```python
from build123d import *

# Parameters (mm, degrees)
SKETCH3_W           = 200
SKETCH3_H           = 50
BOSS_EXTRUDE2_DEPTH = 1
SKETCH4_R           = 2
BOSS_EXTRUDE3_DEPTH = 2


with BuildPart() as part:
    # Sketch3 → Boss-Extrude2 (new, symmetric)
    with BuildSketch(Plane(origin=(0, 0, 0), x_dir=(1, 0, 0), z_dir=(0, 1, 0))):
        Rectangle(SKETCH3_W, SKETCH3_H)
    extrude(amount=BOSS_EXTRUDE2_DEPTH, both=True)

    # Sketch4 → Boss-Extrude3 (add)
    # profile 1 of 2: a face of its own
    with BuildSketch(Plane.XY.offset(25)):
        with BuildLine():
            Line((100, -1), (90, -1))
            Line((90, -1), (90, 21))
            ThreePointArc((90, 21), (95, 26), (100, 21))
            Line((100, 21), (100, -1))
        make_face()
        with Locations((95, 21)):
            Circle(SKETCH4_R, mode=Mode.SUBTRACT)
    # profile 2 of 2: a face of its own
    with BuildSketch(Plane.XY.offset(25)):
        with BuildLine():
            Line((-90, -1), (-90, 21))
            ThreePointArc((-90, 21), (-95, 26), (-100, 21))
            Line((-100, 21), (-100, -1))
            Line((-100, -1), (-90, -1))
        make_face()
        with Locations(Location((-95, 21, 0), (0, 0, 180))):
            Circle(SKETCH4_R, mode=Mode.SUBTRACT)
    extrude(amount=BOSS_EXTRUDE3_DEPTH)


solid = part.part
```
Here's how the part is built. I have some questions about the finished solid (model axes, mm). A direction names the side the tool comes from. Round coordinates to 2 decimals unless told otherwise and drop trailing zeros. Write each loop counter-clockwise with the first axis right and the second up, starting at its lowest first coordinate (ties: lowest second). Pieces come first, ordered by that corner, then holes. Notation, with made-up numbers: M 21.5,-17 L 33.5,-17 A34 ccw 33.5,16 Z; hole C 52.25,88 d11. An arc over 180 degrees is marked long. Answer as CSV lines item,"result". Start each with the question number.
1. Suppose I cut it at D-D on z = 5. Write out the boundary of the cut face in (x, y), then the cut area to 3 significant figures.
2. Suppose I cut it at A-A on y = 15. Write out the boundary of the cut face in (x, z).
3. Thinking about a two-plate mould opening in X: for faces 3 (the cylindrical face through (96.908, 21.601, 25.986)), 4 (the flat face through (-1, 1, 0)), 5 (the flat face through (100, 0, 9)), 6 (the cylindrical face through (95, 26, 26)), which applies, released by +X, released by -X, zero draft, split by the parting line, or undercut?
4. On a 3-axis mill with a long thin cutter (end or side, diameter ignored), from which of +Z, -Z, +X, -X, +Y, -Y can I reach the whole of each face in a straight line? I mean faces 1 (the flat face through (1, -1, 1)), 2 (the flat face through (-95, 14, 25)). Say none if no direction works.
5. I need wall thicknesses on probe 1 along Y at (x, z) = (-95, 25.8); probe 2 along Y at (x, z) = (-1, -6). Which ranges of each line are inside material? Lowest first, please.
6. I'm going to push flat-ended pins straight in: pin 1 Ø5 at (x, y) = (95.5, 18.5) entering from -Z; pin 2 Ø10 at (x, z) = (-71.5, -17) entering from +Y; pin 3 Ø2 at (x, y) = (24.5, 0) entering from +Z. Where does each tip first touch, or does it pass through?
7. Suppose I cut it at B-B on x = 95. Write out the boundary of the cut face in (y, z), then the cut area to 3 significant figures.
8. Suppose I cut it at C-C on x = -84. Write out the boundary of the cut face in (y, z).
Check result:
1,outline,"M -100,-1 L 100,-1 L 100,1 L -100,1 Z"
1,area,"400 mm2"
2,outline,"M -100,25 L -90,25 L -90,27 L -100,27 Z; M 90,25 L 100,25 L 100,27 L 90,27 Z"
3,face 3,"undercut"
3,face 4,"zero draft"
3,face 5,"released by +X"
3,face 6,"undercut"
4,face 1,"+Z, -Z, +X, -X, -Y"
4,face 2,"-Z, +X, -X, +Y"
5,probe 1,"y = -1 to 19, 23 to 26"
5,probe 2,"y = -1 to 1"
6,pin 1,"stops at z = 25"
6,pin 2,"stops at y = 1"
6,pin 3,"stops at z = 25"
7,outline,"M -1,-25 L 1,-25 L 1,25 L 19,25 L 19,27 L -1,27 Z; M 23,25 L 26,25 L 26,27 L 23,27 Z"
7,area,"146 mm2"
8,outline,"M -1,-25 L 1,-25 L 1,25 L -1,25 Z"
